Build history of the part. All positions in model axes, mm. Round coordinates to 2 decimals unless told otherwise and drop trailing zeros. Loops run counter-clockwise (first coordinate to the right, second up) from the corner with the lowest first, then second, coordinate; pieces in that order, holes last.
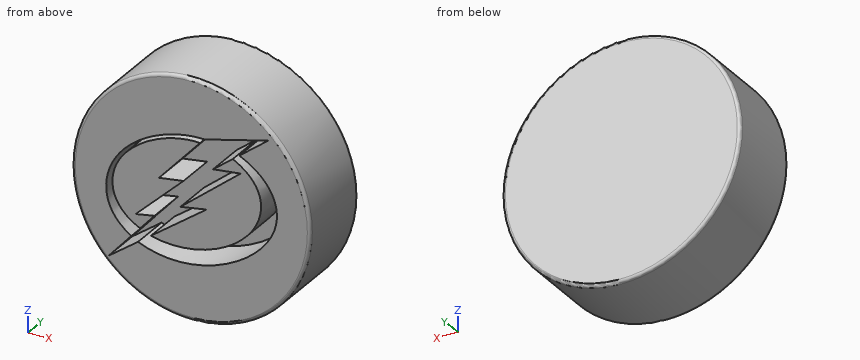
from build123d import *

# Parameters (mm, degrees)
F3_R     = 38.1
F4_DEPTH = 12.7
F5_DEPTH = 12.7
F6_R     = 1


with BuildPart() as f4:
    # F3 (on Front) → F4 (new body, symmetric)
    with BuildSketch(Plane.XZ):
        Circle(F3_R)
    extrude(amount=F4_DEPTH, both=True)

    # F0 (on Front) + F1 (on Front) + F2 (on Front) → F5 (cut)
    with BuildSketch(Plane.XZ):
        Polygon((-11.8081336841, -8.5378140211), (-26.464993082, -25.2349018068), (4.8301340017, -1.8485224727), (-3.5016993061, -3.3492420334), (15.7506130636, 12.5613436103), (6.9332248531, 11.4183481783), (24.5728250593, 25.4238694906), (4.1189347394, 19.9994817376), (-10.358533822, 3.8266193587), (-2.5237547234, 5.047195591), (-17.8205184639, -9.6808085218), align=None)
    with BuildSketch(Plane.XZ):
        with BuildLine():
            Line((-19.0900918096, -17.018487677), (-16.3832232356, -13.7969218194))
            add(Edge.make_bspline(
                [(-16.3832232356, -13.7969218194), (-25.3736051563, -9.473731392), (-29.0905786368, 8.1572549104), (-7.3840054694, 19.1332485124), (2.8318234254, 18.4940695763)],
                knots=[0, 0, 0, 0, 0.4527371046, 1, 1, 1, 1], degree=3))
            Line((2.8318234254, 18.4940695763), (4.588526208, 20.0228095055))
            add(Edge.make_bspline(
                [(-19.0900918096, -17.018487677), (-28.620544821, -11.2098539248), (-29.5136057934, 10.2947418894), (-6.1136707664, 20.5405261368), (4.588526208, 20.0228095055)],
                knots=[0, 0, 0, 0, 0.4639479817, 1, 1, 1, 1], degree=3))
        make_face()
    with BuildSketch(Plane.XZ):
        with BuildLine():
            add(Edge.make_bspline(
                [(-13.784956187, -14.9299576879), (-0.5538631669, -18.623918621), (24.9938380842, -8.3206427927), (23.5522668809, 11.1457686871), (13.0951637402, 16.5083874017)],
                knots=[0, 0, 0, 0, 0.5594726936, 1, 1, 1, 1], degree=3))
            Line((-13.784956187, -14.9299576879), (-17.4717549235, -18.0134642869))
            add(Edge.make_bspline(
                [(-17.4717549235, -18.0134642869), (-0.7163750913, -25.6539166477), (35.1580871339, -8.4938520858), (26.0995104909, 13.357847929), (14.8380147293, 18.3182712644)],
                knots=[0, 0, 0, 0, 0.5723759264, 1, 1, 1, 1], degree=3))
            Line((14.8380147293, 18.3182712644), (13.0951637402, 16.5083874017))
        make_face()
    extrude(amount=F5_DEPTH, mode=Mode.SUBTRACT)

    # F6
    f6_edges = [f4.edges().sort_by_distance(p)[0] for p in [
        (-38.1, -12.7, 0),
        (-38.1, 12.7, 0),
    ]]
    fillet(f6_edges, radius=F6_R)


solid = f4.part
(1) Pin check, flat tips, straight feed: P1, Ø4, axis at x = -25.5, y = 7.5, coming from the +Z side; P2, Ø8, axis at y = -4.5, z = -8, coming from the +X side; P3, Ø8, axis at y = 8.5, z = 27, coming from the +X side. Stop position of each tip, or through.
Responses:
P1: stops at z = 29.99
P2: stops at x = 37.89
P3: stops at x = 30.37
(2) Slice it at B-B on y = 10.25. List the corners of the cut face in (x, z), plus the area to 3 significant figures.
Responses:
outline: circle Ø76.2 at (0, 0)
area: 4,560 mm2
(3) Probe line 1 (Z direction, x = -17, y = -4); line 2 (Z direction, x = 4.5, y = -10.25); line 3 (Z direction, x = -18, y = -0.75). List the from-to ranges inside material, lowest first.
Responses:
line 1: z = -34.1 to -18.22, -13.49 to -9.52, -8.89 to 12.34, 13.63 to 34.1
line 2: z = -37.83 to -19.52, -14.58 to -2.1, -1.91 to 3.26, 20.1 to 37.83
line 3: z = -33.58 to -18.91, -12.94 to 11.57, 12.91 to 33.58
(4) Slice it at A-A on y = -3.5. Count the separate pieces of the cut face and the enclosed holes in it, plus the area to 3 significant figures.
Responses:
separate pieces: 3
enclosed holes: 1
area: 3,680 mm2
